Here's the drawing with two shaded views (mm, measured from the low corner). I have some questions. A direction names the side the tool comes from. Give positions to 0.01 mm unless a question says otherwise; leave off trailing zeros. Loops run counter-clockwise (first coordinate to the right, second up) from the corner with the lowest first, then second, coordinate; pieces in that order, holes last. Notation, with made-up numbers: (84.5, 24) -> (91.5, 24) arc R12 ccw to (91.5, 29) -> close; hole circle Ø5 at (58.5, -16.75). An arc over 180 degrees is marked (long way). Put each result on its own line as item: value.
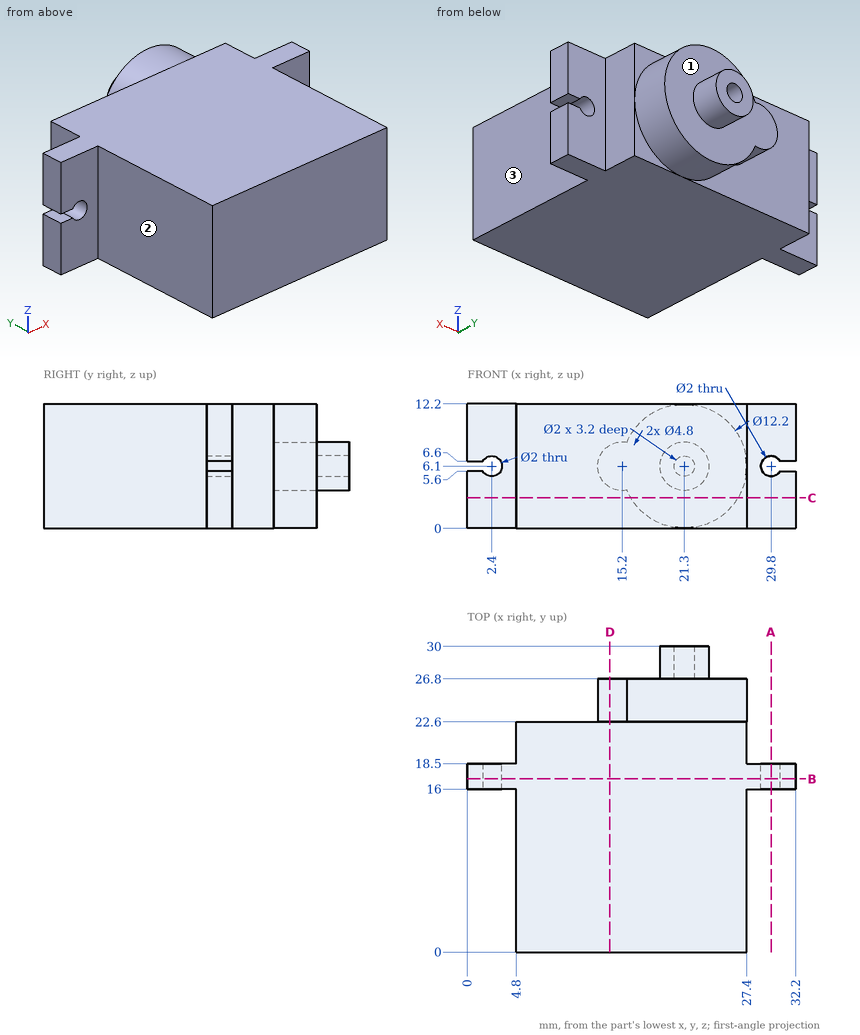
1. If we section it at B-B (y = 17): List the corners of the cut face in (x, z) for me, then the cut area to 3 significant figures.
Recorded:
outline: (0, 0) -> (32.2, 0) -> (32.2, 5.6) -> (30.67, 5.6) arc R1 cw (long way) to (30.67, 6.6) -> (32.2, 6.6) -> (32.2, 12.2) -> (0, 12.2) -> (0, 6.6) -> (1.53, 6.6) arc R1 cw (long way) to (1.53, 5.6) -> (0, 5.6) -> close
area: 384 mm^2
2. I'm going to push flat-ended pins straight in: pin 1 (5 mm diameter, centred on x = 24, z = 4, fed in from +Y); pin 2 (3 mm diameter, centred on y = 13, z = 2, fed in from -X); pin 3 (4 mm diameter, centred on x = 3.5, z = 6.5, fed in from +Y); pin 4 (2.5 mm diameter, centred on x = 2.4, z = 6.1, fed in from +Y). Where does each tip first touch, or does it pass through?
Recorded:
pin 1: stops at y = 30
pin 2: stops at x = 4.8
pin 3: stops at y = 22.6
pin 4: stops at y = 18.5
3. I need wall thicknesses on line 1 (X direction, y = 28.85, z = 6.1); line 2 (Y direction, x = 20.5, z = 9.25); line 3 (X direction, y = 10.5, z = 7.5). Which ranges of each line are inside material? Lowest first, please.
Recorded:
line 1: x = 18.9 to 20.3, 22.3 to 23.7
line 2: y = 0 to 26.8
line 3: x = 4.8 to 27.4
4. If we section it at C-C (z = 3): List the corners of the cut face in (x, y) for me.
Recorded:
outline: (0, 16) -> (4.8, 16) -> (4.8, 0) -> (27.4, 0) -> (27.4, 16) -> (32.2, 16) -> (32.2, 18.5) -> (27.4, 18.5) -> (27.4, 22.6) -> (26.55, 22.6) -> (26.55, 26.8) -> (16.05, 26.8) -> (16.05, 22.6) -> (4.8, 22.6) -> (4.8, 18.5) -> (0, 18.5) -> close
5. If we section it at D-D (x = 14): List the corners of the cut face in (y, z) for me.
Recorded:
outline: (0, 0) -> (22.6, 0) -> (22.6, 4.02) -> (26.8, 4.02) -> (26.8, 8.18) -> (22.6, 8.18) -> (22.6, 12.2) -> (0, 12.2) -> close
6. If we section it at A-A (x = 29.8): List the corners of the cut face in (y, z) for me.
Recorded:
outline: (16, 0) -> (18.5, 0) -> (18.5, 5.1) -> (16, 5.1) -> close; (16, 7.1) -> (18.5, 7.1) -> (18.5, 12.2) -> (16, 12.2) -> close
7. For the marked faces 1, 2 and 3, which set-ups out of +Z, -Z, +X, -X, +Y, -Y let a thin tool reach every point of the face, with its end or its side?
Recorded:
face 1: +Y
face 2: +Z, -Z, -X, -Y
face 3: +Z, -Z, +X, -Y
